Read the model definition and answer for the solid it produces. Units are mm, in the model's axes. A direction names the side the tool comes from. Coordinates: 2 decimals unless noted, no trailing zeros. Write each loop counter-clockwise with the first axis right and the second up, starting at its lowest first coordinate (ties: lowest second). Pieces come first, ordered by that corner, then holes. Notation, with made-up numbers: (9.25, 40) -> (27.25, 40) arc R29 cw to (27.25, 67) -> close; hole circle Ø8 at (73, -21). An arc over 180 degrees is marked (long way). Write item = value, one per line. Start each with the question number.
1) Find the intervals of material crossed by line 1 along Y through (x, z) = (0, 16.65); line 2 along Z through (x, y) = (-6, 9.5); line 3 along Z through (x, y) = (-1.75, 14), in increasing order. Write a range as from..to.
2) Section D-D (z = 22) is taken. Determine the outline of the cut face in (x, y).
3) A tool of negligible diameter and unlimited length cuts with its end or side. For faces 1 (the face through (0, -11, 25)), 2 (the face through (-2.601, -11.715, 21.549)), 3 (the face through (3, -11, 18)), from which of +Z, -Z, +X, -X, +Y, -Y can it reach the whole face along a straight path? Write none if from no direction.
4) Flat-ended cylindrical pins translate along their axes: pin 1 Ø8 at (y, z) = (14.5, 17.5) entering from -X; pin 2 Ø3 at (x, z) = (-4.5, 21.5) entering from -Y; pin 3 Ø1.5 at (x, z) = (-2, 19) entering from +Y. Find the tip coordinate at first contact, or state that the pin passes through.
5) Section A-A (x = 0) is taken. Determine the outline of the cut face in (y, z).
6) Section B-B (y = -2) is taken. Determine the outline of the cut face in (x, z) (3 decimals), plus the area to 3 significant figures.
7) Section C-C (x = -4.75) is taken. Determine the outline of the cut face in (y, z), plus the area to 3 significant figures.
Solid Edge part; units mm, degrees
sketch "Sketch1" plane through (0, 0, 0) normal (0, 0, 1) x (1, 0, 0)
  circle A0 centre (0, 0) radius 9
  circle A1 centre (0, 0) radius 11
extrude "Protrusion1" add sketch "Sketch1" along normal blind 25
sketch "Sketch2" plane through (0, 0, 20) normal (0, 0, 1) x (1, 0, 0)
  circle A0 centre (0, 22) radius 1.5
  line L0 (-3.389, 22.8746) -> (-7.1308, 8.3756)
  arc A1 (-7.1308, 8.3756) -> (7.1308, 8.3756) centre (0, 0) cw
  line L1 (7.1308, 8.3756) -> (3.389, 22.8746)
  arc A2 (3.389, 22.8746) -> (-3.389, 22.8746) centre (0, 22) ccw
extrude "Extrusionsausprägung_3" add sketch "Sketch2" against normal blind 5
sketch "Sketch3" plane through (0, 0, 0) normal (0, -1, 0) x (1, 0, 0)
  line L0 (-11, 17.5) -> (0, 10)
  line L1 (0, 10) -> (11, 17.5)
  dimension "D1" = 11
extrude "Cutout1" cut sketch "Sketch3" along normal through all and the other way through all material side at (-5.5282, 0, 13.7087)
fillet "Verrundung_2" radius 4 2 edges at (0, -10, 10) (0, 10, 10)
sketch "Sketch4" plane through (0, 0, 25) normal (0, 0, 1) x (1, 0, 0)
  circle A0 centre (0, 0) radius 12
  circle A1 centre (0, 0) radius 9
extrude "Extrusionsausprägung_4" add sketch "Sketch4" against normal blind 7
sketch "Sketch5" plane through (0, 0, 25) normal (0, 0, 1) x (1, 0, 0)
  circle A0 centre (0, 0) radius 10.5
extrude "Extrusionsausschnitt_7" cut sketch "Sketch5" against normal blind 6
properties part number "094" material "Aluminiumlegierung:3.0205, Al 99.0, EN-AW 1200"
Answer key:
q1.line_1 = -11..-9, 9..20.5, 23.5..25.5
q1.line_2 = 15..25
q1.line_3 = 15..20
q2.outline = circle Ø24 at (0, 0); hole circle Ø21 at (0, 0)
q3.face_1 = +Z, +X, -X, +Y, -Y
q3.face_2 = +Z
q3.face_3 = -Z
q4.pin_1 = -6.58
q4.pin_2 = -11.62
q4.pin_3 = 25.27
q5.outline = (-12, 18) -> (-11, 18) -> (-11, 10.84) -> (-9, 10.84) -> (-9, 19) -> (-10.5, 19) -> (-10.5, 25) -> (-12, 25) -> close; (9, 10.84) -> (11, 10.84) -> (11, 15) -> (20.5, 15) -> (20.5, 20) -> (12, 20) -> (12, 25) -> (10.5, 25) -> (10.5, 19) -> (9, 19) -> close; (23.5, 15) -> (25.5, 15) -> (25.5, 20) -> (23.5, 20) -> close
q6.outline = (-11.832, 18) -> (-10.817, 18) -> (-10.817, 17.375) -> (-8.775, 15.983) -> (-8.775, 19) -> (-10.308, 19) -> (-10.308, 25) -> (-11.832, 25) -> close; (8.775, 15.983) -> (10.817, 17.375) -> (10.817, 18) -> (11.832, 18) -> (11.832, 25) -> (10.308, 25) -> (10.308, 19) -> (8.775, 19) -> close
q6.area = 29.8 mm^2
q7.outline = (-11.02, 18) -> (-9.92, 18) -> (-9.92, 13.24) -> (-7.64, 13.24) -> (-7.64, 19) -> (-9.36, 19) -> (-9.36, 25) -> (-11.02, 25) -> close; (7.64, 13.24) -> (9.92, 13.24) -> (9.92, 15) -> (17.6, 15) -> (17.6, 20) -> (11.02, 20) -> (11.02, 25) -> (9.36, 25) -> (9.36, 19) -> (7.64, 19) -> close
q7.area = 84.5 mm^2
